```python
from build123d import *

# Parameters (mm, degrees)
SKETCH_1_W          = 150
SKETCH_1_H          = 150
EXTRUDE_1_DEPTH     = 3
SKETCH_2_W          = 150
SKETCH_2_H          = 150
SKETCH_2_W_2        = 144
SKETCH_2_H_2        = 144
EXTRUDE_2_DEPTH     = 40
SKETCH_3_R          = 4
SKETCH_3_R_2        = 1.65
CUT_EXTRUDE_1_DEPTH = 174.130008953


with BuildPart() as part:
    # 草图1 → 凸台-拉伸1 (new body)
    with BuildSketch(Plane(origin=(0, 0, 0), x_dir=(1, 0, 0), z_dir=(0, 1, 0))):
        Rectangle(SKETCH_1_W, SKETCH_1_H)
    extrude(amount=EXTRUDE_1_DEPTH)

    # 草图2 → 凸台-拉伸2 (add)
    with BuildSketch(Plane(origin=(0, 3, 0), x_dir=(1, 0, 0), z_dir=(0, 1, 0))):
        Rectangle(SKETCH_2_W, SKETCH_2_H)
        Rectangle(SKETCH_2_W_2, SKETCH_2_H_2, mode=Mode.SUBTRACT)
    extrude(amount=EXTRUDE_2_DEPTH)

    # 草图3 → 切除-拉伸1 (cut, through all)
    with BuildSketch(Plane(origin=(75, 0, 0), x_dir=(0, 0, -1), z_dir=(1, 0, 0))):
        with Locations((-20.1, 43)):
            Circle(SKETCH_3_R)
        with Locations((-0.1, 23)):
            Circle(SKETCH_3_R_2)
        with Locations((-40.1, 23)):
            Circle(SKETCH_3_R_2)
    extrude(amount=-CUT_EXTRUDE_1_DEPTH, mode=Mode.SUBTRACT)


solid = part.part
```
Geometry check sheet. Reference: the model listing, model coordinates, mm. A direction names the side the tool comes from. Round coordinates to 2 decimals unless told otherwise and drop trailing zeros. Loops run counter-clockwise (first coordinate to the right, second up) from the corner with the lowest first, then second, coordinate; pieces in that order, holes last. Notation, with made-up numbers: (-26, -26) -> (30, -26) arc R7 cw to (30, -22) -> close; hole circle Ø4 at (55.5, 31.25). An arc over 180 degrees is marked (long way). Use a Markdown table: item, result.
(1) Sectioned sample at C-C (z = -25). Enter the section's corners in (x, y).
Calculated:
| item | result |
|---|---|
| outline | (-75, 0) -> (75, 0) -> (75, 43) -> (72, 43) -> (72, 3) -> (-72, 3) -> (-72, 43) -> (-75, 43) -> close |
(2) Sectioned sample at A-A (y = 19). Enter the section's corners in (x, z), then the cut area to 3 significant figures.
Calculated:
| item | result |
|---|---|
| outline | (-75, -75) -> (75, -75) -> (75, 75) -> (-75, 75) -> close; hole (-72, -72) -> (72, -72) -> (72, 72) -> (-72, 72) -> close |
| area | 1,760 mm² |
(3) Mould release check, pull along Y, two halves, no side actions. Record for faces 3 (the flat face through (-23, 43, 74)), 4 (the flat face through (-1, 21, -75)), 5 (the cylindrical face through (73.521, 24.636, 0.315)), 6 (the cylindrical face through (73.521, 24.115, 41.316)): released by +Y, released by -Y, zero draft, split by the parting line, or undercut.
Calculated:
| item | result |
|---|---|
| face 3 | released by +Y |
| face 4 | zero draft |
| face 5 | undercut |
| face 6 | undercut |
(4) Sectioned sample at B-B (x = -21.5). Enter the section's corners in (y, z), then the cut area to 3 significant figures.
Calculated:
| item | result |
|---|---|
| outline | (0, -75) -> (43, -75) -> (43, -72) -> (3, -72) -> (3, 72) -> (43, 72) -> (43, 75) -> (0, 75) -> close |
| area | 690 mm² |
(5) Scan lines: probe 1 along Y at (x, z) = (-73.25, 40.1); probe 2 along Z at (x, y) = (-46.5, 28.5). Record each from-to range of solid material in increasing order.
Calculated:
| item | result |
|---|---|
| probe 1 | 0 to 21.35, 24.65 to 43 |
| probe 2 | -75 to -72, 72 to 75 |
(6) Go/stop test with flat-tipped pins: P1, Ø5, axis at x = -2.5, z = 17.5, coming from the +Y side; P2, Ø2, axis at y = 23, z = 0.1, coming from the -X side. Record where each tip stops, or that it passes through.
Calculated:
| item | result |
|---|---|
| P1 | y = 3 |
| P2 | through |
(7) Set-up check for faces 1 (the flat face through (-1, 23, 72)), 2 (the flat face through (-34, 43, -74)): record each of +Z, -Z, +X, -X, +Y, -Y from which the full face is reachable in a straight line by a thin tool's end or side.
Calculated:
| item | result |
|---|---|
| face 1 | +Y |
| face 2 | +Z, -Z, +X, -X, +Y |
